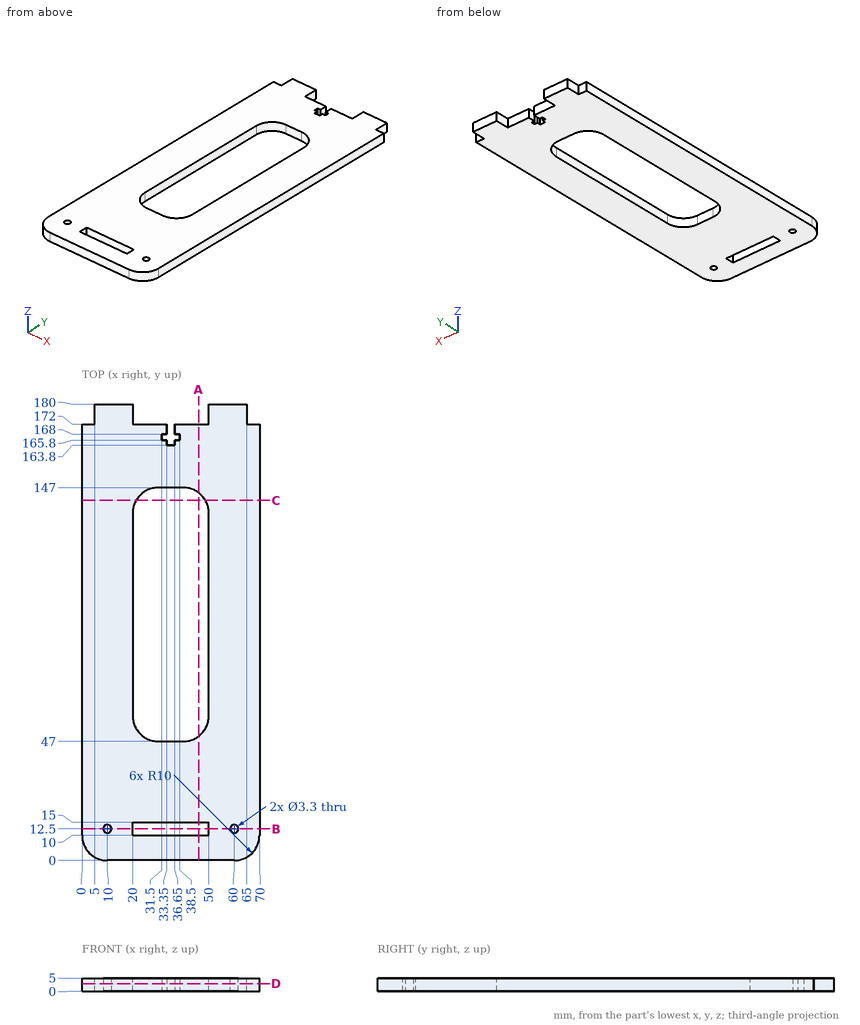
The drawing under review shows one solid part. Ordinate dimensions are in mm from its lowest x, y, z. Coordinates: 2 decimals unless noted, no trailing zeros. Order: outer loops, then holes, each group sorted by start corner. A loop starts at its lowest first (then second) coordinate and runs counter-clockwise, first axis right, second up. Notation, with made-up numbers: (54.5, 45) -> (96.5, 45) arc R21 cw to (96.5, 78) -> close; hole circle Ø8 at (8, 5.5). An arc over 180 degrees is marked (long way). Answer in a Markdown table with one row per item. Add a question column.
Item 1: We need section D-D on z = 3. Give the number of separate pieces and of enclosed holes in the cut face, plus the area to 3 significant figures.
Item 2: Clearance check with flat-ended pins moving along their axes: pin 1 (0.6 mm diameter, centred on x = 37.5, z = 1.5, fed in from +Y); pin 2 (1.5 mm diameter, centred on y = 178, z = 1.5, fed in from +X). State where each tip first meets the part, or that it passes through.
Item 3: We need section B-B on y = 12.5. Write out the cut boundary in (x, z).
Item 4: We need section A-A on x = 46. Write out the cut boundary in (y, z).
Item 5: To check wall thickness, follow probe 1 along Y at (x, z) = (36, 1.8); probe 2 along Y at (x, z) = (40.5, 0.55); probe 3 along Y at (x, z) = (60, 3.9). State the ranges of each line that lie inside material, in increasing order.
Item 6: We need section C-C on y = 142. Write out the cut boundary in (x, z).
Final values:
| question | item | result |
|---|---|---|
| 1 | separate pieces | 1 |
| 1 | enclosed holes | 4 |
| 1 | area | 9,120 mm2 |
| 2 | pin 1 | stops at y = 172 |
| 2 | pin 2 | stops at x = 65 |
| 3 | outline | (0, 0) -> (8.35, 0) -> (8.35, 5) -> (0, 5) -> close; (11.65, 0) -> (20, 0) -> (20, 5) -> (11.65, 5) -> close; (50, 0) -> (58.35, 0) -> (58.35, 5) -> (50, 5) -> close; (61.65, 0) -> (70, 0) -> (70, 5) -> (61.65, 5) -> close |
| 4 | outline | (0, 0) -> (10, 0) -> (10, 5) -> (0, 5) -> close; (15, 0) -> (49, 0) -> (49, 5) -> (15, 5) -> close; (145, 0) -> (172, 0) -> (172, 5) -> (145, 5) -> close |
| 5 | probe 1 | y = 0 to 10, 15 to 47, 147 to 163.8 |
| 5 | probe 2 | y = 0 to 10, 15 to 47.01, 146.99 to 172 |
| 5 | probe 3 | y = 0 to 10.85, 14.15 to 180 |
| 6 | outline | (0, 0) -> (21.34, 0) -> (21.34, 5) -> (0, 5) -> close; (48.66, 0) -> (70, 0) -> (70, 5) -> (48.66, 5) -> close |
